Work out the finished part from the listing and answer in its coordinate system (mm). A direction names the side the tool comes from. Coordinates: 2 decimals unless noted, no trailing zeros. Order: outer loops, then holes, each group sorted by start corner. A loop starts at its lowest first (then second) coordinate and runs counter-clockwise, first axis right, second up.
```python
from build123d import *

# Parameters (mm, degrees)
BOSS_EXTRUDE1_DEPTH = 5
FILLET1_R           = 10
SKETCH2_R           = 1.25
CUT_EXTRUDE1_DEPTH  = 53.440442409


with BuildPart() as part:
    # Sketch1 → Boss-Extrude1 (new body)
    with BuildSketch(Plane(origin=(0, 0, 0), x_dir=(1, 0, 0), z_dir=(0, 1, 0))):
        with BuildLine():
            Line((0, 10), (0, 50))
            Line((0, 50), (-15, 50))
            Line((-15, 50), (-15, 11.480705826))
            Line((-15, 11.480705826), (-9.360265408, -3.519294174))
            ThreePointArc((-9.360265408, -3.519294174), (8.221707297, -5.692409782), (0, 10))
        make_face()
    extrude(amount=BOSS_EXTRUDE1_DEPTH)

    # Fillet1
    fillet1_edges = [part.edges().sort_by_distance(p)[0] for p in [
        (0, 2.5, -10),
    ]]
    fillet(fillet1_edges, radius=FILLET1_R)

    # Sketch2 → Cut-Extrude1 (cut, through all)
    with BuildSketch(Plane(origin=(0, 5, 0), x_dir=(1, 0, 0), z_dir=(0, 1, 0))):
        with Locations(Location((0, 0, 0), (0, 0, 270))):
            Circle(SKETCH2_R)
    extrude(amount=-CUT_EXTRUDE1_DEPTH, mode=Mode.SUBTRACT)


solid = part.part
```
1. A flat-ended cylindrical pin translates along its axis: pin 1 (2.5 mm diameter, centred on y = 1.5, z = -36.5, fed in from +X). Find the tip coordinate at first contact, or state that the pin passes through.
2. The part is cut by section C-C (z = -24). Determine the outline of the cut face in (x, y).
3. The part is cut by section A-A (y = 1.55). Determine the outline of the cut face in (x, z).
4. Consider probe 1 along X at (y, z) = (3.35, -34); probe 2 along X at (y, z) = (3.65, 0); probe 3 along X at (y, z) = (4, -11). Determine where each line is inside the solid, lowest interval first.
5. The part is cut by section B-B (z = 0). Determine the outline of the cut face in (x, y).
6. The part is cut by section D-D (x = -12). Determine the outline of the cut face in (y, z).
7. For faces 1 (the flat face through (-12.22, 2.46, -4.09)), 2 (the flat face through (0, 2, -33)), determine the directions among +Z, -Z, +X, -X, +Y, -Y from which every point of the face is accessible in a straight line to the end or side of a thin tool.
Worked out:
1. pin 1: stops at x = 0
2. outline: (-15, 0) - (0, 0) - (0, 5) - (-15, 5) - close
3. outline: (-15, -50) - (0, -50) - (0, -17.32) arc R10 cw to (5, -8.66) arc R10 ccw (long way) to (-9.36, 3.52) - (-15, -11.48) - close; hole circle Ø2.5 at (0, 0)
4. probe 1: x = -15 to 0
4. probe 2: x = -10.68 to -1.25, 1.25 to 10
4. probe 3: x = -14.82 to 2.25
5. outline: (-10.68, 0) - (-1.25, 0) - (-1.25, 5) - (-10.68, 5) - close; (1.25, 0) - (10, 0) - (10, 5) - (1.25, 5) - close
6. outline: (0, -50) - (5, -50) - (5, -3.5) - (0, -3.5) - close
7. face 1: +Z, -X, +Y, -Y
7. face 2: -Z, +X, +Y, -Y
